Could you check a few things on this model? Use its own coordinates, in mm. A direction names the side the tool comes from. Round coordinates to 2 decimals unless told otherwise and drop trailing zeros. Loops run counter-clockwise (first coordinate to the right, second up) from the corner with the lowest first, then second, coordinate; pieces in that order, holes last. Notation, with made-up numbers: (-5, 69) -> (45, 69) arc R25 ccw to (45, 91) -> close; hole circle Ø4 at (-6, 53). An arc over 180 degrees is marked (long way). Put each result on its own line as item: value. Start each with the question number.
1. If we mould it in two halves opening along Z, with no side actions, what happens to faces 1 (the flat face through (-50, -8, 0)), 2 (the flat face through (-1, -8, -26)), 3 (the flat face through (51.5, 2, 0)), 4 (the flat face through (-53.5, -8, 0))? For each: pulls with the +Z half, pulls with the -Z half, needs draft (parallel to the pull), parting line crosses it, or undercut.
2. Imagine slicing it at B-B, the plane x = -47.5. Please give me the cut outline in (y, z).
3. I'm going to push flat-ended pins straight in: P1, Ø5, axis at x = 2, y = -4.5, coming from the +Z side; P2, Ø7.5, axis at y = -9, z = 4.5, coming from the -X side; P3, Ø5, axis at x = -1, y = 2.5, coming from the +Z side; P4, Ø8, axis at x = 17.5, z = -16, coming from the +Y side. Where does each tip first touch, or does it pass through?
4. I need wall thicknesses on line 1 (X direction, y = -10.75, z = 17.5); line 2 (X direction, y = 1, z = -1.5); line 3 (Z direction, x = -22.5, y = -3.25). Which ranges of each line are inside material? Lowest first, please. Write a range as [from, to].
5. Which directions (+Z, -Z, +X, -X, +Y, -Y) give clear straight access to the entire face, cutting with the end or side of a thin tool? Please do faces 5 (the cylindrical face through (-58.57, 0.99, 31)), 6 (the flat face through (0, -1, -23)), 7 (the flat face through (-1, -8, 22.5)).
6. Imagine slicing it at C-C, the plane y = -9.75. Please give me the cut outline in (x, z), and give its area (3 significant figures).
7. Imagine slicing it at A-A, the plane z = -0.5. Please give me the cut outline in (x, y), and give its area (3 significant figures).
```python
from build123d import *

# Parameters (mm, degrees)
SKETCH1_W           = 100
SKETCH1_H           = 45
BOSS_EXTRUDE1_DEPTH = 5
SKETCH2_W           = 107
SKETCH2_H           = 52
SKETCH2_W_2         = 100
SKETCH2_H_2         = 45
BOSS_EXTRUDE2_DEPTH = 16
FILLET1_R           = 3
SKETCH3_W           = 103
SKETCH3_H           = 48
SKETCH3_W_2         = 100
SKETCH3_H_2         = 45
CUT_EXTRUDE1_DEPTH  = 6


with BuildPart() as part:
    # Sketch1 → Boss-Extrude1 (new body)
    with BuildSketch(Plane(origin=(0, 0, 0), x_dir=(1, 0, 0), z_dir=(0, 1, 0))):
        with BuildLine():
            Line((-55, -32.5), (55, -32.5))
            ThreePointArc((55, -32.5), (58.535533906, -31.035533906), (60, -27.5))
            Line((60, -27.5), (60, 27.5))
            ThreePointArc((60, 27.5), (58.535533906, 31.035533906), (55, 32.5))
            Line((55, 32.5), (-55, 32.5))
            ThreePointArc((-55, 32.5), (-58.535533906, 31.035533906), (-60, 27.5))
            Line((-60, 27.5), (-60, -27.5))
            ThreePointArc((-60, -27.5), (-58.535533906, -31.035533906), (-55, -32.5))
        make_face()
        Rectangle(SKETCH1_W, SKETCH1_H, mode=Mode.SUBTRACT)
    extrude(amount=BOSS_EXTRUDE1_DEPTH)

    # Sketch2 → Boss-Extrude2 (add)
    with BuildSketch(Plane.XZ):
        Rectangle(SKETCH2_W, SKETCH2_H)
        Rectangle(SKETCH2_W_2, SKETCH2_H_2, mode=Mode.SUBTRACT)
    extrude(amount=BOSS_EXTRUDE2_DEPTH)

    # Fillet1
    fillet1_edges = [part.edges().sort_by_distance(p)[0] for p in [
        (58.535533906, 5, 31.035533906),
        (60, 5, 0),
        (58.535533906, 5, -31.035533906),
        (0, 5, -32.5),
        (-58.535533906, 5, -31.035533906),
        (-60, 5, 0),
        (-58.535533906, 5, 31.035533906),
        (0, 5, 32.5),
    ]]
    fillet(fillet1_edges, radius=FILLET1_R)

    # Sketch3 → Cut-Extrude1 (cut)
    with BuildSketch(Plane(origin=(0, 5, 0), x_dir=(1, 0, 0), z_dir=(0, 1, 0))):
        Rectangle(SKETCH3_W, SKETCH3_H)
        Rectangle(SKETCH3_W_2, SKETCH3_H_2, mode=Mode.SUBTRACT)
    extrude(amount=-CUT_EXTRUDE1_DEPTH, mode=Mode.SUBTRACT)


solid = part.part
```
Entries:
1. face 1: undercut
1. face 2: pulls with the -Z half
1. face 3: undercut
1. face 4: needs draft
2. outline: (-16, -26) -> (0, -26) -> (0, -32.5) -> (2, -32.5) arc R3 ccw to (5, -29.5) -> (5, -24) -> (-1, -24) -> (-1, -22.5) -> (-16, -22.5) -> close; (-16, 22.5) -> (-1, 22.5) -> (-1, 24) -> (5, 24) -> (5, 29.5) arc R3 ccw to (2, 32.5) -> (0, 32.5) -> (0, 26) -> (-16, 26) -> close
3. P1: z = 26
3. P2: x = -53.5
3. P3: z = 32.5
3. P4: through
4. line 1: [-53.5, -50], [50, 53.5]
4. line 2: [-60, -51.5], [51.5, 60]
4. line 3: [-26, -22.5], [22.5, 26]
5. face 5: +Z, -X, +Y, -Y
5. face 6: +Y
5. face 7: +Y, -Y
6. outline: (-53.5, -26) -> (53.5, -26) -> (53.5, 26) -> (-53.5, 26) -> close; hole (-50, -22.5) -> (50, -22.5) -> (50, 22.5) -> (-50, 22.5) -> close
6. area: 1,060 mm^2
7. outline: (-60, 0) -> (-53.5, 0) -> (-53.5, -16) -> (-50, -16) -> (-50, -1) -> (-51.5, -1) -> (-51.5, 5) -> (-57, 5) arc R3 ccw to (-60, 2) -> close; (50, -16) -> (53.5, -16) -> (53.5, 0) -> (60, 0) -> (60, 2) arc R3 ccw to (57, 5) -> (51.5, 5) -> (51.5, -1) -> (50, -1) -> close
7. area: 190 mm^2
